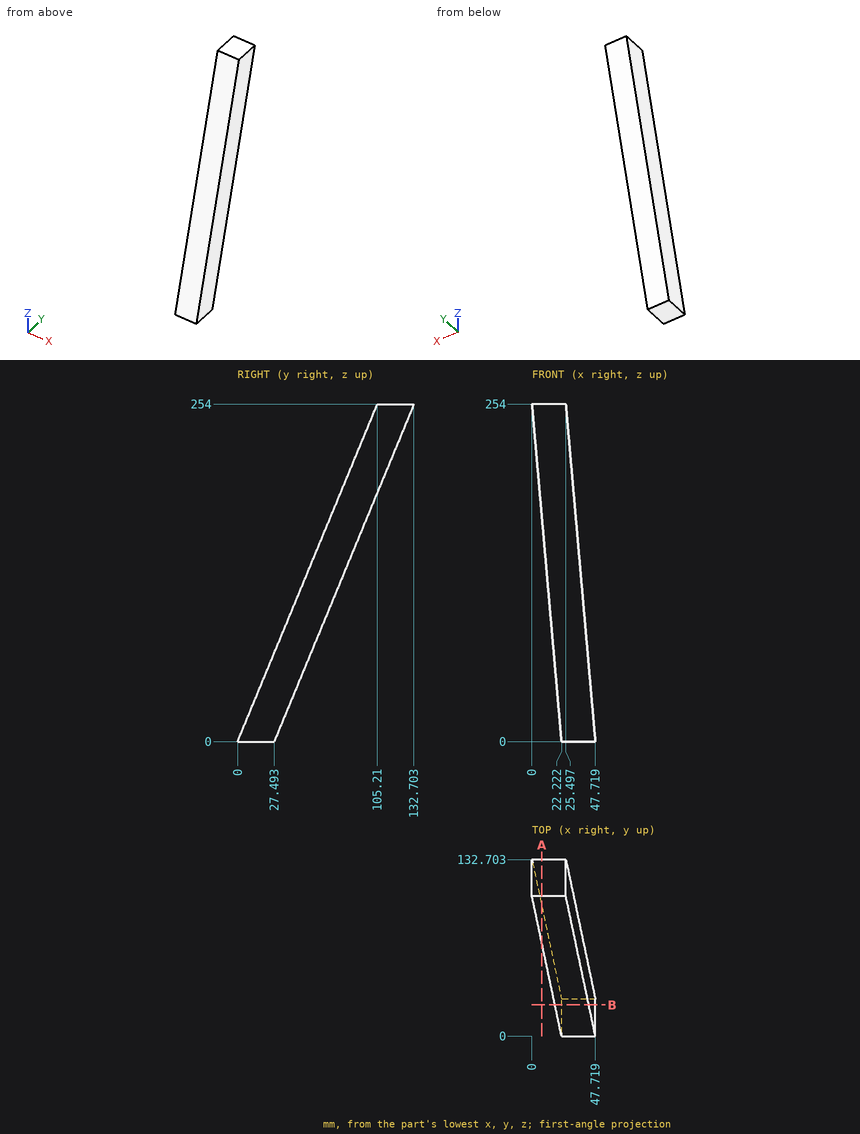
Check sheet for the drawn part. Datum: minimum x, y, z corner. Units: mm. Coordinates: 2 decimals unless noted, no trailing zeros. Order: outer loops, then holes, each group sorted by start corner. A loop starts at its lowest first (then second) coordinate and runs counter-clockwise, first axis right, second up. Notation, with made-up numbers: (56.25, -39) - (106.25, -39) arc R22 ccw to (106.25, -28) - close; hole circle Ø7 at (62, 31.25). An arc over 180 degrees is marked (long way). Return JSON: item names as keys, results as strings.
(1) Go/stop test with flat-tipped pins: pin 1 (10 mm diameter, centred on y = 53.5, z = 89.5, fed in from -X); pin 2 (1 mm diameter, centred on x = 14, y = 79, fed in from +Z); pin 3 (1.5 mm diameter, centred on y = 65.5, z = 131.5, fed in from +X). Record where each tip stops, or that it passes through.
Filled sheet:
{"pin 1": "stops at x = 13.95", "pin 2": "stops at z = 191.93", "pin 3": "stops at x = 36.28"}
(2) Thickness scan on line 1 along Z through (x, y) = (20.5, 76) (1 decimal); line 2 along Y through (x, z) = (34.5, 87.5); line 3 along Y through (x, z) = (21.5, 61.5) (1 decimal). Record the ranges inside material, lowest first.
Filled sheet:
{"line 1": "z = 117.1 to 183.5", "line 2": "y = 36.24 to 63.74", "line 3": "y = 25.5 to 53"}
(3) Section check A-A, the plane x = 7.5. Record the cut outline in (y, z) (1 decimal), and give its area (3 significant figures).
Filled sheet:
{"outline": "(69.7, 168.3) - (97.2, 168.3) - (132.7, 254) - (105.2, 254) - close", "area": "2,360 mm^2"}
(4) Section check B-B, the plane y = 23.5. Record the cut outline in (x, z), and give its area (3 significant figures).
Filled sheet:
{"outline": "(17.26, 56.73) - (22.22, 0) - (47.72, 0) - (42.76, 56.73) - close", "area": "1,450 mm^2"}
